Autodesk Inventor part; units mm, degrees
ref_plane "YZ Plane" through (0, 0, 0) normal (1, 0, 0) x (0, 1, 0)
ref_plane "XZ Plane" through (0, 0, 0) normal (0, 1, 0) x (-1, 0, 0)
ref_plane "XY Plane" through (0, 0, 0) normal (0, 0, 1) x (1, 0, 0)
sketch "スケッチ1" plane through (0, 0, 0) normal (0, 0, 1) x (1, 0, 0)
  line L0 (0, 0) -> (15, 0)
  line L1 (15, 0) -> (15, 15)
  line L2 (15, 15) -> (0, 15)
  line L3 (0, 15) -> (0, 0)
  dimension "d0" = 15
  dimension "d1" = 15
extrude "押し出し1" add sketch "スケッチ1" along normal blind 120
sketch "スケッチ2" plane through (0, 15, 0) normal (0, 1, 0) x (1, 0, 0)
  line L0 (0, 0) -> (0, -120)
  line L1 (15, 0) -> (0, 0)
  line L2 (15, -120) -> (0, -120)
  point P0 (7.5, -10)
  point P1 (7.5, -20)
  point P2 (7.5, -110)
  point P3 (7.5, -100)
  dimension "d4" = 7.5
  dimension "d5" = 10
  dimension "d6" = 10
  dimension "d7" = 7.5
  dimension "d8" = 10
  dimension "d9" = 7.5
  dimension "d10" = 10
  dimension "d11" = 7.5
hole "穴1" at (7.5, 15, 10) at (7.5, 15, 20) at (7.5, 15, 110) at (7.5, 15, 100) direction (0, -1, 0) diameter 3.2 end through all
sketch "スケッチ3" plane through (0, 0, 120) normal (0, 0, 1) x (1, 0, 0)
  line L0 (1.5, 13.5) -> (13.5, 13.5)
  line L1 (13.5, 13.5) -> (13.5, 1.5)
  line L2 (13.5, 1.5) -> (1.5, 1.5)
  line L3 (1.5, 1.5) -> (1.5, 13.5)
  line L4 (15, 15) -> (0, 15)
  line L5 (0, 15) -> (0, 0)
  dimension "d19" = 12
  dimension "d20" = 12
  dimension "d21" = 1.5
  dimension "d22" = 1.5
extrude "押し出し2" cut sketch "スケッチ3" against normal blind 200
properties part number "射出_角柱9" material "アルミニウム 6061"
Can you work these out from the model? Positions are in its coordinate system, mm. A direction names the side the tool comes from. Round coordinates to 2 decimals unless told otherwise and drop trailing zeros. Write each loop counter-clockwise with the first axis right and the second up, starting at its lowest first coordinate (ties: lowest second). Pieces come first, ordered by that corner, then holes. Notation, with made-up numbers: M 89,-33.5 L 129,-33.5 A27 ccw 129,-9.5 Z; hole C -29.5,13 d6. An arc over 180 degrees is marked long. Use a Markdown table: item, result.
Item 1: Which directions (+Z, -Z, +X, -X, +Y, -Y) give clear straight access to the entire face, cutting with the end or side of a thin tool? Please do faces 5 (the face through (8.47, 14.24, 18.73)), 6 (the face through (1.5, 7, 61)).
Found:
| item | result |
|---|---|
| face 5 | +Y, -Y |
| face 6 | +Z, -Z |
Item 2: We'd pull the mould along Z, two halves only. Please class faces 1 (the face through (7, 13.5, 61)), 2 (the face through (8.47, 0.74, 108.73)), 3 (the face through (7.43, 0.74, 98.4)), 4 (the face through (14, 8, 120)): released by +Z, released by -Z, zero draft, split by the parting line, or undercut.
Found:
| item | result |
|---|---|
| face 1 | zero draft |
| face 2 | undercut |
| face 3 | undercut |
| face 4 | released by +Z |
Item 3: For pin 1 Ø3 at (x, z) = (7.5, 100) entering from +Y (1 decimal), with a flat end and sliding along its axis, tell me the tip position at first contact or that it passes through.
Found:
| item | result |
|---|---|
| pin 1 | passes through |
Item 4: I want a section at A-A (x = 10.75). List the corners of the cut face in (y, z) for me.
Found:
| item | result |
|---|---|
| outline | M 0,0 L 1.5,0 L 1.5,120 L 0,120 Z; M 13.5,0 L 15,0 L 15,120 L 13.5,120 Z |
Item 5: I want a section at B-B (z = 25). List the corners of the cut face in (x, y) for me, and give its area (3 significant figures).
Found:
| item | result |
|---|---|
| outline | M 0,0 L 15,0 L 15,15 L 0,15 Z; hole M 1.5,1.5 L 13.5,1.5 L 13.5,13.5 L 1.5,13.5 Z |
| area | 81.0 mm2 |
Item 6: If I drill on line 1 along Z through (x, y) = (7.5, 1); line 2 along Y through (x, z) = (5, 65); line 3 along X through (y, z) = (1.1, 100), over which ranges is the centre line in solid material (lowest first)? Write a range as [from, to].
Found:
| item | result |
|---|---|
| line 1 | z = [0, 8.4], [11.6, 18.4], [21.6, 98.4], [101.6, 108.4], [111.6, 120] |
| line 2 | y = [0, 1.5], [13.5, 15] |
| line 3 | x = [0, 5.9], [9.1, 15] |
